The model under review builds one solid part; all positions refer to its coordinate system, in mm. A direction names the side the tool comes from. Round coordinates to 2 decimals unless told otherwise and drop trailing zeros. Order: outer loops, then holes, each group sorted by start corner. A loop starts at its lowest first (then second) coordinate and runs counter-clockwise, first axis right, second up. Notation, with made-up numbers: M 42.25,2.5 L 85.25,2.5 A15 cw 85.25,26.5 Z; hole C -22,86.25 d10. An arc over 180 degrees is marked long. Answer as a JSON object with one key per item and string values. Group by question number.
1. Add section B-B on x = 25. State the section outline as (y, z) points.
2. Add section C-C on x = 20.5. State the section outline as (y, z) points.
3. Machinability: for faces 5 (the face through (25.56, 4.27, 0.56)), 6 (the face through (8.121, -16.353, 3.631)), which of the approach directions +Z, -Z, +X, -X, +Y, -Y give a long, thin tool a straight path to every point of the face, cutting with its end or side? Answer none if there is none.
4. Mouldability with a two-part tool opening along Z and no side actions: class faces 1 (the face through (18.94, -14.58, 3.24)), 2 (the face through (14.79, -10.17, 17.96)), 3 (the face through (14.79, -10.46, -17.79)), 4 (the face through (15, 20.638, 0)) as released by +Z, released by -Z, zero draft, split by the parting line, or undercut.
5. Clearance check with flat-ended pins moving along their axes: P1, Ø10, axis at y = 0, z = 0, coming from the -X side; P2, Ø5, axis at x = 22, z = 12.5, coming from the -Y side; P3, Ø5, axis at x = 3.5, y = -11.5, coming from the -Z side; P4, Ø4, axis at x = 7.5, y = -10, coming from the -Z side. State where each tip first meets the part, or that it passes through.
6. To check wall thickness, follow probe 1 along Y at (x, z) = (19.5, 0); probe 2 along Y at (x, z) = (11.75, 0); probe 3 along X at (y, z) = (-12.5, 9). State the ranges of each line that lie inside material, in increasing order. Write a range as [from, to].
```python
from build123d import *

# Parameters (mm, degrees)
EXTRUDE1_DEPTH = 29.972
CHAMFER1_SIZE  = 0.508
CHAMFER3_SIZE  = 0.762
CHAMFER4_SIZE  = 0.762
FILLET1_R      = 0.508


with BuildPart() as part:
    # Sketch1 → Extrude1 (new body)
    with BuildSketch(Plane(origin=(0, 0, 0), x_dir=(0, 0, -1), z_dir=(1, 0, 0))):
        Polygon((11.91506618, 20.6375), (-11.91506618, 20.6375), (-23.830132361, 0), (-11.91506618, -20.6375), (11.91506618, -20.6375), (23.830132361, 0), align=None)
    extrude(amount=EXTRUDE1_DEPTH)

    # Sketch2 → Cut-Revolve1 (revolve, cut)
    with BuildSketch(Plane.XY, mode=Mode.PRIVATE) as cut_revolve1_sk:
        Polygon((0, 16.7513), (0, 0), (29.972, 0), (29.972, 8.255), (29.718, 8.255), (29.718, 4.953), (29.591, 4.926005317), (28.970294683, 4.3053), (22.2504, 4.3053), (21.4884, 5.0673), (21.4884, 14.9352), (16.4592, 14.9352), (16.4592, 16.7513), align=None)
    revolve(cut_revolve1_sk.sketch.rotate(Axis((0, 0, 0), (1, 0, 0)), 270), axis=Axis((0, 0, 0), (1, 0, 0)), mode=Mode.SUBTRACT)  # turned: the seam where the file's is

    # Chamfer1
    chamfer1_edges = [part.edges().sort_by_distance(p)[0] for p in [
        (0, 0, 16.7513),
    ]]
    chamfer(chamfer1_edges, length=CHAMFER1_SIZE)

    # Chamfer3
    chamfer3_edges = [part.edges().sort_by_distance(p)[0] for p in [
        (0, -10.31875, -17.872599271),
        (0, -20.6375, 0),
        (0, -10.31875, 17.872599271),
        (0, 10.31875, 17.872599271),
        (0, 20.6375, 0),
        (0, 10.31875, -17.872599271),
    ]]
    chamfer(chamfer3_edges, length=CHAMFER3_SIZE)

    # Chamfer4
    chamfer4_edges = [part.edges().sort_by_distance(p)[0] for p in [
        (29.972, 10.31875, 17.872599271),
        (29.972, -10.31875, 17.872599271),
        (29.972, -20.6375, 0),
        (29.972, -10.31875, -17.872599271),
        (29.972, 10.31875, -17.872599271),
        (29.972, 20.6375, 0),
    ]]
    chamfer(chamfer4_edges, length=CHAMFER4_SIZE)

    # Fillet1
    fillet1_edges = [part.edges().sort_by_distance(p)[0] for p in [
        (16.4592, 0, 16.7513),
    ]]
    fillet(fillet1_edges, radius=FILLET1_R)


solid = part.part
```
Recorded:
{
 "1": {"outline": "M -20.64,-11.92 L 0,-23.83 L 20.64,-11.92 L 20.64,11.92 L 0,23.83 L -20.64,11.92 Z; hole C 0,0 d8.61"},
 "2": {"outline": "M -20.64,-11.92 L 0,-23.83 L 20.64,-11.92 L 20.64,11.92 L 0,23.83 L -20.64,11.92 Z; hole C 0,0 d29.87"},
 "3": {"face 5": "+X, -X", "face 6": "-X"},
 "4": {"face 1": "undercut", "face 2": "released by +Z", "face 3": "released by -Z", "face 4": "zero draft"},
 "5": {"P1": "stops at x = 21.56", "P2": "stops at y = -20.64", "P3": "stops at z = -18.63", "P4": "stops at z = -19.21"},
 "6": {"probe 1": "y = [-20.64, -14.94], [14.94, 20.64]", "probe 2": "y = [-20.64, -16.75], [16.75, 20.64]", "probe 3": "x = [16.46, 29.97]"}
}
